Build history of the part. All positions in model axes, mm. Face numbers are marked on the shaded views. A direction names the side the tool comes from. Give positions to 0.01 mm unless a question says otherwise; leave off trailing zeros. Write each loop counter-clockwise with the first axis right and the second up, starting at its lowest first coordinate (ties: lowest second). Pieces come first, ordered by that corner, then holes. Notation, with made-up numbers: (22, -24.5) -> (47, -24.5) arc R21 ccw to (47, 1.5) -> close; hole circle Ø4 at (39.25, -20.5). An arc over 180 degrees is marked (long way). Put each result on its own line as item: value. Start each with the question number.
Item 1: Slice it at B-B, the plane x = 1. List the corners of the cut face in (y, z), plus the area to 3 significant figures.
Item 2: Drill centre lines: line 1 along Z through (x, y) = (0, 5); line 2 along Z through (x, y) = (0, 7.5); line 3 along X through (y, z) = (8.75, 2.5). Where is each one in solid material? Low to high.
Item 3: Slice it at D-D, the plane x = -0.5. Give the number of separate pieces and of enclosed holes in the cut face, plus the area to 3 significant figures.
Item 4: Slice it at C-C, the plane y = 3. List the corners of the cut face in (x, z), plus the area to 3 significant figures.
Item 5: Flat gauge pins, fed straight in: pin 1 Ø3 at (y, z) = (10.5, 5) entering from +X; pin 2 Ø2 at (x, z) = (-1, 14.5) entering from -Y; pin 3 Ø2 at (x, z) = (2.5, 13.5) entering from -Y. Where does each tip first touch, or does it go through?
Item 6: Tool access for the marked faces 5 and 6: list every direction of +Z, -Z, +X, -X, +Y, -Y with a clear straight run to the whole face (end or side of a thin tool).
Item 7: Two-plate mould, pull along Y, no slides. Class the marked faces 1, 2, 3 and 4: pulls with the +Y half, pulls with the -Y half, needs draft (parallel to the pull), parting line crosses it, or undercut.
Item 8: Slice it at A-A, the plane z = 3. List the corners of the cut face in (x, y).
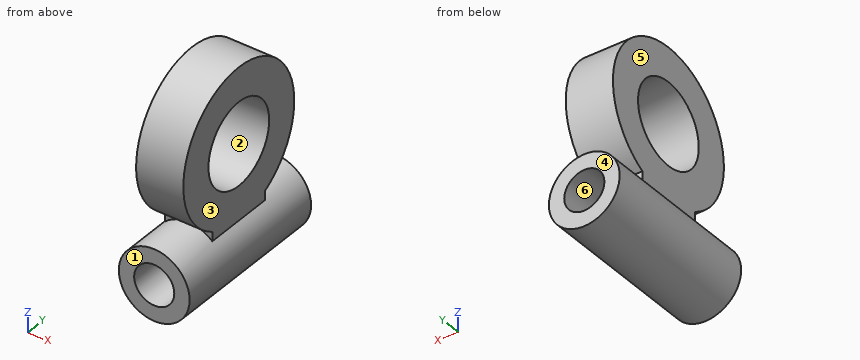
Autodesk Fusion 360 part; units mm, degrees
sketch "Sketch1" plane through (0, 0, 0) normal (0, 1, 0) x (1, 0, 0)
  circle A0 centre (0, -3) radius 3
  circle A1 centre (0, -3) radius 1.7
  dimension "d1" = 3.4
extrude "Extrude1" add sketch "Sketch1" along normal blind 14
sketch "Sketch2" plane through (0, 0, 0) normal (0, 0, 1) x (1, 0, 0)
ref_plane "WorkPlane1" through (0, 0, 6) normal (0, 0, 1) x (1, 0, 0)
sketch "Sketch3" plane through (0, 0, 6) normal (0, 0, 1) x (1, 0, 0)
  line L0 (-2, 10.0294) -> (2, 10.0294)
  line L1 (2, 10.0294) -> (2, 3.9745)
  line L2 (2, 3.9745) -> (-2, 3.9745)
  line L3 (-2, 3.9745) -> (-2, 10.0294)
extrude "Extrude2" add sketch "Sketch3" against normal blind 1
ref_plane "WorkPlane2" through (-2, 0, 0) normal (1, 0, 0) x (0, 1, 0)
sketch "Sketch4" plane through (-2, 0, 0) normal (1, 0, 0) x (0, 1, 0)
  circle A0 centre (7.0273, 11.6383) radius 6.3914
  circle A1 centre (7.0273, 11.6383) radius 3.5
  dimension "d8" = 7
extrude "Extrude3" add sketch "Sketch4" along normal blind 4
Values follow:
1. outline: (0, 0.17) -> (14, 0.17) -> (14, 1.63) -> (0, 1.63) -> close; (0, 4.37) -> (14, 4.37) -> (14, 5.83) -> (10.03, 5.83) -> (10.03, 6) arc R6.39 ccw (long way) to (4.02, 6) -> (3.97, 6) -> (3.97, 5.83) -> (0, 5.83) -> close; hole circle Ø7 at (7.03, 11.64)
1. area: 129 mm2
2. line 1: 0 to 1.3, 4.7 to 8.79, 14.49 to 17.7
2. line 2: 0 to 1.3, 4.7 to 8.17, 15.11 to 18.01
2. line 3: -2.96 to -1.62, 1.62 to 2.96
3. separate pieces: 2
3. enclosed holes: 1
3. area: 124 mm2
4. outline: circle Ø6 at (0, 3); (-2, 6.68) -> (2, 6.68) -> (2, 16.6) -> (-2, 16.6) -> close; hole circle Ø3.4 at (0, 3)
4. area: 58.9 mm2
5. pin 1: x = 2.96
5. pin 2: y = 0.91
5. pin 3: y = 0.71
6. face 5: +Z, -X, +Y, -Y
6. face 6: +Y, -Y
7. face 1: pulls with the -Y half
7. face 2: undercut
7. face 3: needs draft
7. face 4: pulls with the +Y half
8. outline: (-3, 0) -> (-1.7, 0) -> (-1.7, 14) -> (-3, 14) -> close; (1.7, 0) -> (3, 0) -> (3, 14) -> (1.7, 14) -> close
